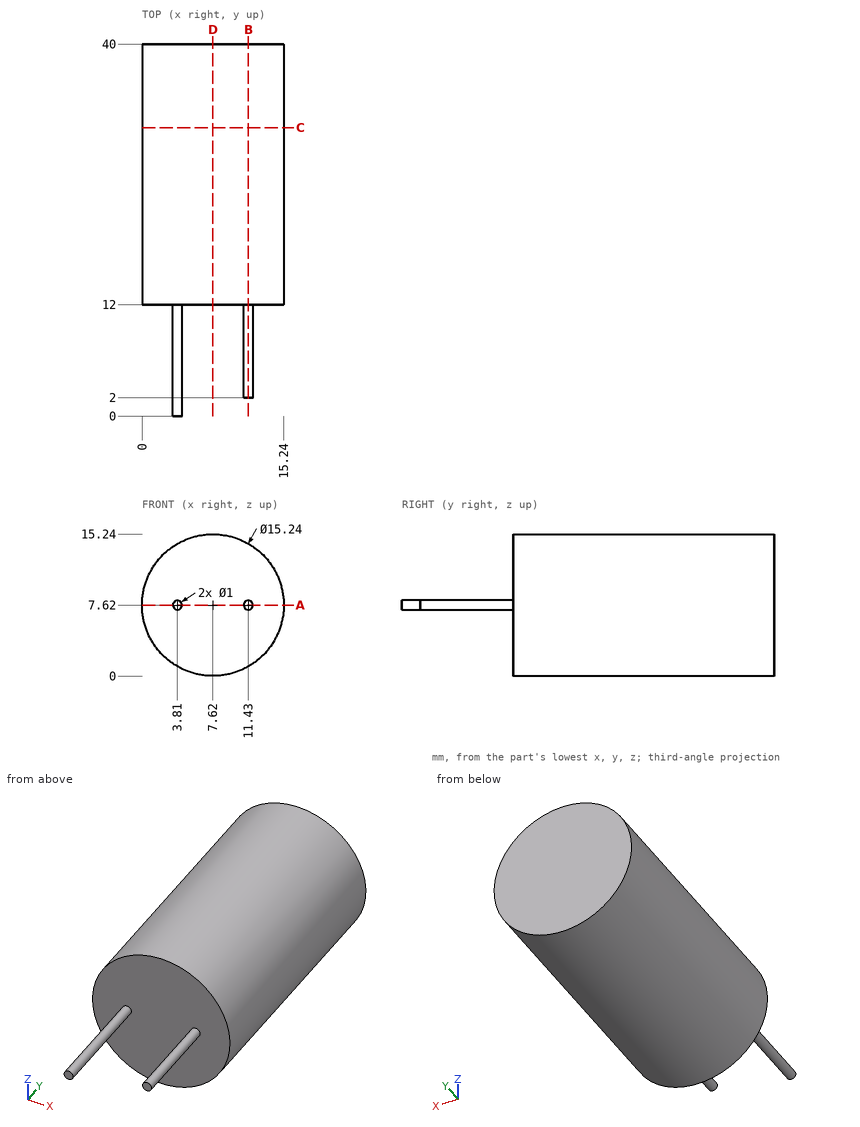
Geometry check sheet. Reference: drawing and pictorial views, mm from the part's lowest x, y, z. Coordinates: 2 decimals unless noted, no trailing zeros. Order: outer loops, then holes, each group sorted by start corner. A loop starts at its lowest first (then second) coordinate and runs counter-clockwise, first axis right, second up.
Item 1: Scan lines: line 1 along Y through (x, z) = (2.25, 9.5); line 2 along Z through (x, y) = (3.75, 2.5); line 3 along Z through (x, y) = (14.25, 38.5). Record each from-to range of solid material in increasing order.
Item 2: Section check C-C (y = 31). Enter the section's corners in (x, z), plus the area to 3 significant figures.
Item 3: Depth check by flat-ended pin: pin 1 (1.5 mm diameter, centred on x = 2, y = 24.5, fed in from -Z); pin 2 (3 mm diameter, centred on x = 3.5, y = 25.5, fed in from +Z); pin 3 (6 mm diameter, centred on x = 13, y = 33.5, fed in from -Z); pin 4 (8 mm diameter, centred on y = 11.5, z = 4.5, fed in from +X). Enter the tip coordinate at first touch or a pass-through.
Item 4: Section check D-D (x = 7.62). Enter the section's corners in (y, z).
Item 5: Section check B-B (x = 11.43). Enter the section's corners in (y, z), plus the area to 3 significant figures.
Item 6: Section check A-A (z = 7.62). Enter the section's corners in (x, y).
Check sheet entries:
1. line 1: y = 12 to 40
1. line 2: z = 7.12 to 8.12
1. line 3: z = 3.86 to 11.38
2. outline: circle Ø15.24 at (7.62, 7.62)
2. area: 182 mm2
3. pin 1: stops at z = 1.76
3. pin 2: stops at z = 14.78
3. pin 3: stops at z = 0.38
3. pin 4: stops at x = 15.24
4. outline: (12, 0) - (40, 0) - (40, 15.24) - (12, 15.24) - close
5. outline: (2, 7.12) - (12, 7.12) - (12, 1.02) - (40, 1.02) - (40, 14.22) - (12, 14.22) - (12, 8.12) - (2, 8.12) - close
5. area: 380 mm2
6. outline: (0, 12) - (3.31, 12) - (3.31, 0) - (4.31, 0) - (4.31, 12) - (10.93, 12) - (10.93, 2) - (11.93, 2) - (11.93, 12) - (15.24, 12) - (15.24, 40) - (0, 40) - close
